Study the drawing (mm; zero at the part's minimum x, y, z) and answer. Give positions to 0.01 mm unless a question says otherwise; leave off trailing zeros. Order: outer loops, then holes, each group sorted by start corner. A loop starts at its lowest first (then second) coordinate and runs counter-clockwise, first axis right, second up. Notation, with made-up numbers: (-22, 43) - (8, 43) arc R28 ccw to (8, 69) - close; hole circle Ø2 at (57.5, 57). An arc over 180 degrees is marked (long way). Write each question's results on one line, items separated by ' | '. Start each with the question number.
1. Section A-A (z = 30) is taken. Give the vertices of the cut face in (x, y), and give its area (4 significant figures).
2. Section C-C (y = 13.5) is taken. Give the vertices of the cut face in (x, z).
3. Section B-B (x = 30) is taken. Give the vertices of the cut face in (y, z).
4. Determine the mould class of the marked faces 1, 2 and 3 for opening direction X: released by +X, released by -X, zero draft, split by the parting line, or undercut.
5. Flat-ended cylindrical pins translate along their axes: pin 1 (8 mm diameter, centred on y = 19, z = 24, fed in from +X); pin 2 (2 mm diameter, centred on x = 42.5, y = 17.5, fed in from +Z); pin 3 (12 mm diameter, centred on y = 13, z = 35.5, fed in from +X); pin 4 (1.9 mm diameter, centred on x = 30, z = 11.8, fed in from -Y). Find the tip coordinate at first contact, or state that the pin passes through.
6. Section D-D (z = 50) is taken. Give the vertices of the cut face in (x, y), and give its area (3 significant figures).
7. Find the intervals of material crossed by L1, parallel to X at y = 18.5, z = 30; L2, parallel to Y at x = 25, z = 14; L3, parallel to Z at x = 40, y = 11.25, in increasing order.
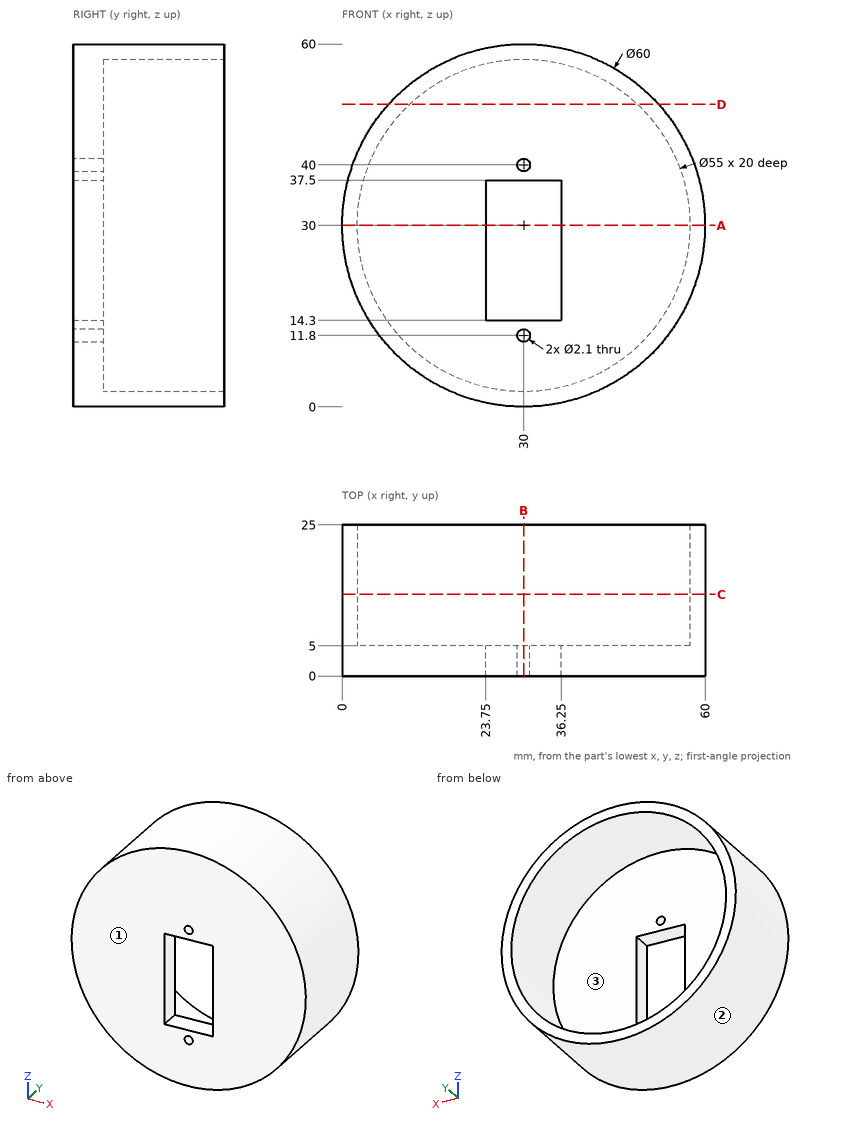
Reported:
1) outline: (0, 0) - (23.75, 0) - (23.75, 5) - (2.5, 5) - (2.5, 25) - (0, 25) - close; (36.25, 0) - (60, 0) - (60, 25) - (57.5, 25) - (57.5, 5) - (36.25, 5) - close | area: 337.5 mm²
2) outline: circle Ø60 at (30, 30); hole circle Ø55 at (30, 30)
3) outline: (0, 0) - (25, 0) - (25, 2.5) - (5, 2.5) - (5, 10.75) - (0, 10.75) - close; (0, 12.85) - (5, 12.85) - (5, 14.3) - (0, 14.3) - close; (0, 37.5) - (5, 37.5) - (5, 38.95) - (0, 38.95) - close; (0, 41.05) - (5, 41.05) - (5, 57.5) - (25, 57.5) - (25, 60) - (0, 60) - close
4) face 1: zero draft | face 2: split by the parting line | face 3: undercut
5) pin 1: x = 59.93 | pin 2: z = 57.71 | pin 3: x = 60 | pin 4: through
6) outline: (7.64, 0) - (52.36, 0) - (52.36, 25) - (48.87, 25) - (48.87, 5) - (11.13, 5) - (11.13, 25) - (7.64, 25) - close | area: 363 mm²
7) L1: 0 to 2.5, 57.5 to 60 | L2: 0 to 5 | L3: 1.72 to 4.38, 55.62 to 58.28
